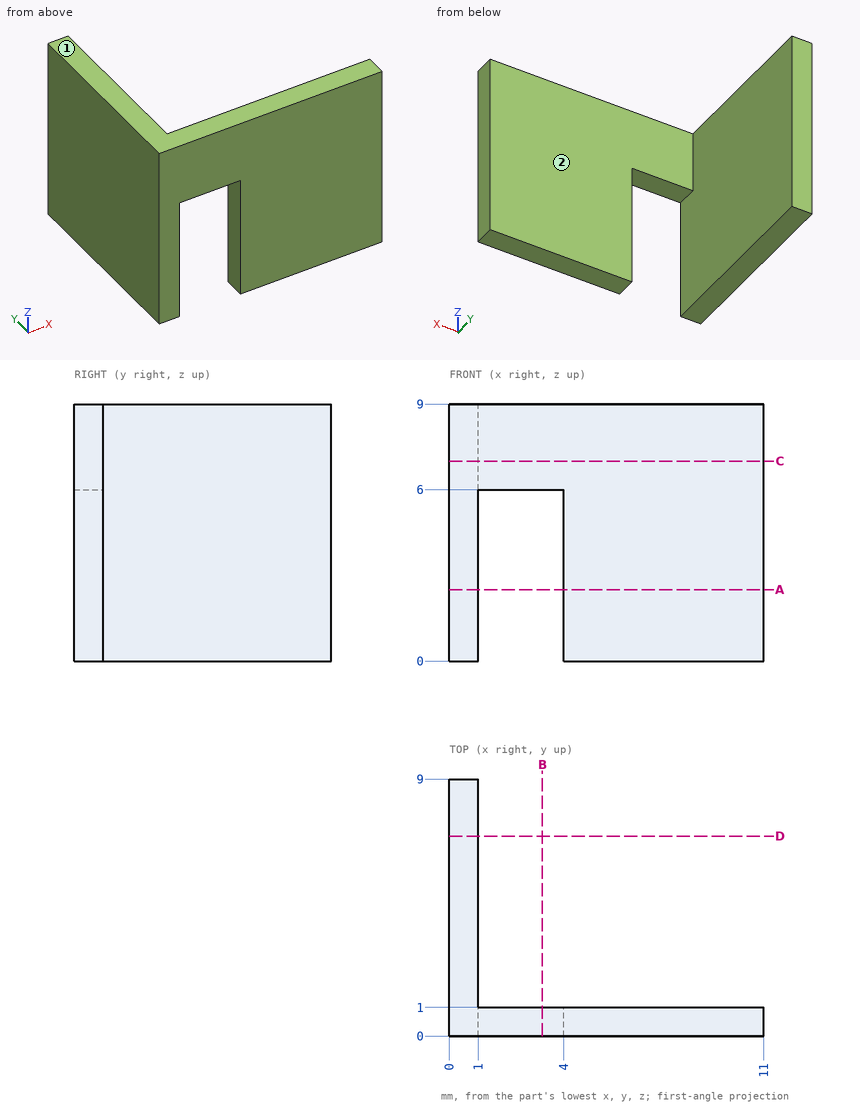
Study the drawing (mm; zero at the part's minimum x, y, z) and answer. A direction names the side the tool comes from. Coordinates: 2 decimals unless noted, no trailing zeros. Write each loop counter-clockwise with the first axis right and the second up, starting at its lowest first coordinate (ties: lowest second). Pieces come first, ordered by that corner, then holes. Notation, with made-up numbers: (42, 12) - (98, 12) arc R23 cw to (98, 37) - close; hole circle Ø10 at (-10.75, 37). An arc over 180 degrees is marked (long way). Return JSON: item names as keys, results as strings. Group by question number.
1. A cutting plane is placed at A-A, the plane z = 2.5. Determine the outline of the cut face in (x, y).
2. A cutting plane is placed at C-C, the plane z = 7. Determine the outline of the cut face in (x, y), plus the area to 3 significant figures.
3. A cutting plane is placed at D-D, the plane y = 7. Determine the outline of the cut face in (x, z).
4. Given pin 1 (4.5 mm diameter, centred on y = 5, z = 4, fed in from +X); pin 2 (3 mm diameter, centred on x = 3.5, y = 4, fed in from -Z), each flat-ended and moving along its own axis, determine where each tip first touches the part or whether it passes through.
5. Which of the six approach directions +Z, -Z, +X, -X, +Y, -Y give full straight-line access (tool end or side, diameter ignored) to the marked faces 1 and 2?
6. Straight lines are drawn through the part: L1, parallel to X at y = 1.5, z = 5.5; L2, parallel to Z at x = 3.25, y = 0.5. For each, find the intervals that lie inside material, in ascending order.
7. A cutting plane is placed at B-B, the plane x = 3.25. Determine the outline of the cut face in (y, z).
Ans:
{
 "1": {"outline": "(0, 0) - (1, 0) - (1, 9) - (0, 9) - close; (4, 0) - (11, 0) - (11, 1) - (4, 1) - close"},
 "2": {"outline": "(0, 0) - (11, 0) - (11, 1) - (1, 1) - (1, 9) - (0, 9) - close", "area": "19.0 mm²"},
 "3": {"outline": "(0, 0) - (1, 0) - (1, 9) - (0, 9) - close"},
 "4": {"pin 1": "x = 1", "pin 2": "through"},
 "5": {"face 1": "+Z, +X, -X, +Y, -Y", "face 2": "+Z, -Z, +X, +Y"},
 "6": {"L1": "0 to 1", "L2": "6 to 9"},
 "7": {"outline": "(0, 6) - (1, 6) - (1, 9) - (0, 9) - close"}
}
